Input: part model. Units: mm. Frame: model coordinates. Face numbers are marked on the shaded views. A direction names the side the tool comes from. Coordinates: 2 decimals unless noted, no trailing zeros. Write each loop counter-clockwise with the first axis right and the second up, starting at its lowest first coordinate (ties: lowest second). Pieces come first, ordered by that corner, then holes. Notation, with made-up numbers: M -31.5,44.25 L 8.5,44.25 A37 ccw 8.5,82.25 Z; hole C -28.75,67 d6. An arc over 180 degrees is marked long. Write each question's results on one line, items separated by ' | '. Start each with the question number.
1. Section query B-B, the plane y = 25. Output: boundary loops of the cut face in (x, z), and give its area (3 significant figures).
2. First-contact query: pin 1 (4 mm diameter, centred on x = -9.5, z = 1, fed in from +Y); pin 2 (1.5 mm diameter, centred on y = -14.5, z = 2.5, fed in from +X); pin 3 (10 mm diameter, centred on x = 0, y = 21.35, fed in from +Z); pin 4 (1 mm diameter, centred on x = 24, z = 1.5, fed in from +Y). Flat tips, straight axial feed; report the tip coordinate or a pass-through.
3. Section query D-D, the plane y = 10. Output: boundary loops of the cut face in (x, z).
4. Ray query, probe 1 along X at (y, z) = (-14.5, 1.75); probe 2 along X at (y, z) = (16, 1.5); probe 3 along X at (y, z) = (-5.5, 4.25). Return the intervals inside material, ascending.
5. Set-up query: the marked faces 1 and 2. Return all of +Z, -Z, +X, -X, +Y, -Y with unobstructed straight access to the full face (end or side cutting, diameter ignored); none if empty.
6. Pull-direction query (Y, two-part tool) for the marked faces 3, 4, 5 and 6; classes: +Y half, -Y half, draft (parallel to the pull), parting line (faces both ways), or undercut.
7. Section query A-A, the plane x = 23.5. Output: boundary loops of the cut face in (y, z), and give its area (3 significant figures).
8. Section query C-C, the plane z = 4. Count the separate pieces of the cut face and the enclosed holes in it, and give its area (3 significant figures).
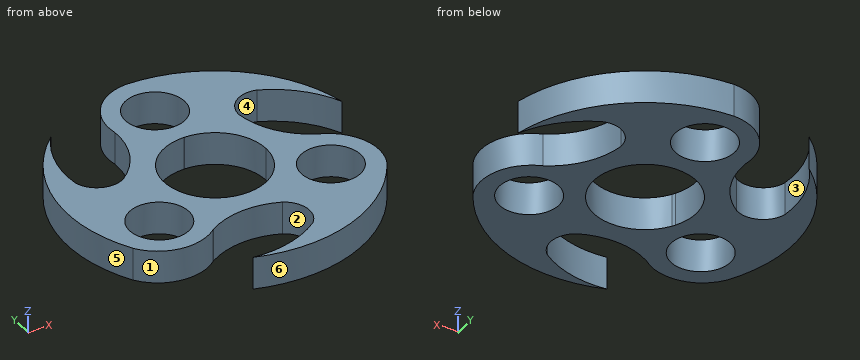
```python
from build123d import *

# Parameters (mm, degrees)
F0_R     = 6.375
F1_DEPTH = 7


with BuildPart() as f1:
    # F0 (on Top) → F1 (new body)
    with BuildSketch(Plane.XY):
        with BuildLine():
            Line((-11.447235, -18.267009), (-11.400234, -18.231657))
            ThreePointArc((-11.400234, -18.231657), (-3.725439, -15.657485), (4.255035, -17.014272))
            ThreePointArc((4.255035, -17.014272), (7.067716, -21.175926), (5.373267, -25.904496))
            ThreePointArc((5.373267, -25.904496), (-1.962484, -29.445234), (-10.082932, -30.084303))
            ThreePointArc((-10.082932, -30.084303), (11.322753, -29.635141), (27.572568, -15.694242))
            ThreePointArc((27.572568, -15.694242), (27.863052, -6.900018), (21.539104, -0.781975))
            Line((21.539104, -0.781975), (21.519969, -0.772949))
            ThreePointArc((21.519969, -0.772949), (15.432301, 4.588143), (12.607275, 12.192104))
            ThreePointArc((12.607275, 12.192104), (14.805032, 16.708784), (19.747318, 17.605634))
            ThreePointArc((19.747318, 17.605634), (26.519114, 12.985588), (31.13793, 6.212954))
            ThreePointArc((31.13793, 6.212954), (20.134618, 24.54515), (0, 31.738163))
            ThreePointArc((0, 31.738163), (-7.913144, 27.634586), (-10.082506, 18.988716))
            Line((-10.082506, 18.988716), (-10.086068, 18.923081))
            ThreePointArc((-10.086068, 18.923081), (-11.71126, 11.025443), (-16.862309, 4.822168))
            ThreePointArc((-16.862309, 4.822168), (-21.872747, 4.467142), (-25.120585, 8.298862))
            ThreePointArc((-25.120585, 8.298862), (-24.519079, 16.422178), (-21.012304, 23.774227))
            ThreePointArc((-21.012304, 23.774227), (-31.326161, 5.011778), (-27.377897, -16.031423))
            ThreePointArc((-27.377897, -16.031423), (-19.93322, -20.676414), (-11.487312, -18.296124))
            Line((-11.487312, -18.296124), (-11.447235, -18.267009))
        make_face()
        with Locations((-18.503675, -10.689365)):
            Circle(F0_R, mode=Mode.SUBTRACT)
        with BuildLine():
            ThreePointArc((0.05941, 10.979839), (7.785009, 7.742999), (10.98, 0))
            ThreePointArc((10.98, 0), (3.012852, -10.558557), (-9.32658, -5.79442))
            ThreePointArc((-9.32658, -5.79442), (-9.51149, -5.485613), (-9.68618, -5.170911))
            ThreePointArc((-9.68618, -5.170911), (-9.423582, 5.63529), (-0.027977, 10.979964))
            ThreePointArc((-0.027977, 10.979964), (0.015717, 10.979989), (0.05941, 10.979839))
        make_face(mode=Mode.SUBTRACT)
        with Locations((18.499237, -10.691927)):
            Circle(F0_R, mode=Mode.SUBTRACT)
        with Locations((0, 21.354815)):
            Circle(F0_R, mode=Mode.SUBTRACT)
    extrude(amount=F1_DEPTH)


solid = f1.part
```
Answer:
1) outline: M -9.45,0 L -5.23,0 L -5.23,7 L -9.45,7 Z; M 5.23,0 L 19.57,0 L 19.57,7 L 5.23,7 Z | area: 130 mm^2
2) pin 1: y = 28.13 | pin 2: x = 28.29 | pin 3: through | pin 4: y = 21.35
3) outline: M -30.11,0 L -25.25,0 L -25.25,7 L -30.11,7 Z; M -12.25,0 L -4.53,0 L -4.53,7 L -12.25,7 Z; M 4.53,0 L 13,0 L 13,7 L 4.53,7 Z; M 29.02,0 L 30.14,0 L 30.14,7 L 29.02,7 Z
4) probe 1: -28.22 to -23.61, -13.39 to 13.39, 23.61 to 28.06 | probe 2: -27.4 to -24.63, -10.22 to -3.46, 3.46 to 14.03, 22.76 to 27.42 | probe 3: -31.24 to -22.21, -14.8 to -9.5, 9.5 to 14.8, 22.2 to 27.18
5) face 1: +Z, -Z, -Y | face 2: +Z, -Z
6) face 3: undercut | face 4: undercut | face 5: parting line | face 6: -Y half
7) outline: M -21.31,0 L -14.65,0 L -14.65,7 L -21.31,7 Z; M -6.74,0 L -1.73,0 L -1.73,7 L -6.74,7 Z; M 15.51,0 L 21.35,0 L 21.35,7 L 15.51,7 Z | area: 123 mm^2
8) separate pieces: 1 | enclosed holes: 4 | area: 1,500 mm^2
